```python
from build123d import *

# Parameters (mm, degrees)
SKETCH2_W           = 57
SKETCH2_H           = 37
BOSS_EXTRUDE1_DEPTH = 1.4
SKETCH1_R           = 1.35
CUT_EXTRUDE2_DEPTH  = 2.4
FILLET1_R           = 2
FILLET2_R           = 2
SKETCH4_R           = 2.5
SKETCH4_R_2         = 1.35
BOSS_EXTRUDE2_DEPTH = 1
CUT_EXTRUDE3_DEPTH  = 2.4


with BuildPart() as part:
    # Sketch2 → Boss-Extrude1 (new body)
    with BuildSketch(Plane(origin=(0, 0, 0), x_dir=(1, 0, 0), z_dir=(0, 1, 0))):
        Polygon((-27.5, -37.5), (-27.5, 37.5), (-22.5, 37.5), (-22.5, 23.5), (13.713455262, 23.5), (24.418761806, 38.487429162), (28.487429162, 35.581238194), (19.85797331, 23.5), (39.5, 23.5), (39.5, -23.5), (19.85797331, -23.5), (28.487429162, -35.581238194), (24.418761806, -38.487429162), (13.713455262, -23.5), (-22.5, -23.5), (-22.5, -37.5), align=None)
        with Locations((6, 0)):
            Rectangle(SKETCH2_W, SKETCH2_H, mode=Mode.SUBTRACT)
    extrude(amount=BOSS_EXTRUDE1_DEPTH)

    # Sketch1 → Cut-Extrude2 (cut, through all)
    with BuildSketch(Plane(origin=(0, 0, 0), x_dir=(1, 0, 0), z_dir=(0, 1, 0))):
        with Locations((-25, 35)):
            Circle(SKETCH1_R)
        with Locations((25, 35)):
            Circle(SKETCH1_R)
        with Locations((25, -35)):
            Circle(SKETCH1_R)
        with Locations((-25, -35)):
            Circle(SKETCH1_R)
        with Locations((-25, 21)):
            Circle(SKETCH1_R)
        with Locations((37, 21)):
            Circle(SKETCH1_R)
        with Locations((37, -21)):
            Circle(SKETCH1_R)
        with Locations((-25, -21)):
            Circle(SKETCH1_R)
    extrude(amount=CUT_EXTRUDE2_DEPTH, mode=Mode.SUBTRACT)

    # Fillet1
    fillet1_edges = [part.edges().sort_by_distance(p)[0] for p in [
        (28.487429162, 0.7, 35.581238194),
        (24.418761806, 0.7, 38.487429162),
        (-22.5, 0.7, 37.5),
        (-27.5, 0.7, 37.5),
        (-27.5, 0.7, -37.5),
        (-22.5, 0.7, -37.5),
        (24.418761806, 0.7, -38.487429162),
        (28.487429162, 0.7, -35.581238194),
    ]]
    fillet(fillet1_edges, radius=FILLET1_R)

    # Fillet2
    fillet2_edges = [part.edges().sort_by_distance(p)[0] for p in [
        (13.713455262, 0.7, 23.5),
        (-22.5, 0.7, 23.5),
        (-22.5, 0.7, -23.5),
        (13.713455262, 0.7, -23.5),
        (19.85797331, 0.7, -23.5),
        (19.85797331, 0.7, 23.5),
        (-22.5, 0.7, 18.5),
        (34.5, 0.7, 18.5),
        (34.5, 0.7, -18.5),
        (-22.5, 0.7, -18.5),
    ]]
    fillet(fillet2_edges, radius=FILLET2_R)

    # Sketch4 → Boss-Extrude2 (add)
    with BuildSketch(Plane(origin=(0, 1.4, 0), x_dir=(1, 0, 0), z_dir=(0, 1, 0))):
        with Locations((37, 21)):
            Circle(SKETCH4_R)
        with Locations((37, 21)):
            Circle(SKETCH4_R_2, mode=Mode.SUBTRACT)
        with Locations((37, -21)):
            Circle(SKETCH4_R)
        with Locations((37, -21)):
            Circle(SKETCH4_R_2, mode=Mode.SUBTRACT)
        with Locations((-25, -21)):
            Circle(SKETCH4_R)
        with Locations((-25, -21)):
            Circle(SKETCH4_R_2, mode=Mode.SUBTRACT)
        with Locations((-25, 21)):
            Circle(SKETCH4_R)
        with Locations((-25, 21)):
            Circle(SKETCH4_R_2, mode=Mode.SUBTRACT)
    extrude(amount=BOSS_EXTRUDE2_DEPTH)

    # Sketch5 → Cut-Extrude3 (cut, through all)
    with BuildSketch(Plane(origin=(0, 1.4, 0), x_dir=(1, 0, 0), z_dir=(0, 1, 0))):
        with BuildLine():
            Line((37, -23.5), (39.5, -23.5))
            Line((39.5, -23.5), (39.5, -21))
            ThreePointArc((39.5, -21), (38.767766953, -22.767766953), (37, -23.5))
        make_face()
        with BuildLine():
            Line((39.5, 21), (39.5, 23.5))
            Line((39.5, 23.5), (37, 23.5))
            ThreePointArc((37, 23.5), (38.767766953, 22.767766953), (39.5, 21))
        make_face()
    extrude(amount=-CUT_EXTRUDE3_DEPTH, mode=Mode.SUBTRACT)


solid = part.part
```
Input: part model. Units: mm. Frame: model coordinates. A direction names the side the tool comes from. Coordinates: 2 decimals unless noted, no trailing zeros. Write each loop counter-clockwise with the first axis right and the second up, starting at its lowest first coordinate (ties: lowest second). Pieces come first, ordered by that corner, then holes.
1) Section A-A on z = 9.5. Output: boundary loops of the cut face in (x, y), and give its area (3 significant figures).
2) Section C-C on x = 25. Output: boundary loops of the cut face in (y, z).
3) Section B-B on x = 1.5. Output: boundary loops of the cut face in (y, z).
4) Set-up query: faces 4 (the cylindrical face through (-23.1, 0.71, 36.93)), 5 (the flat face through (-23.9, 2.4, -19.9)), 6 (the cylindrical face through (-21.93, 0.71, -17.9)), 7 (the flat face through (24.684, 0.69, 30.257)), 8 (the cylindrical face through (-23.1, 0.71, -36.93)). Return all of +Z, -Z, +X, -X, +Y, -Y with unobstructed straight access to the full face (end or side cutting, diameter ignored); none if empty.
5) Mould query, pull axis X, two halves, no side actions, for faces 1 (the cylindrical face through (-26.93, 0.71, 36.9)), 2 (the flat face through (4, 0, 19)), 3 (the cylindrical face through (25.62, 0.69, 36.2)). Classes: pulls with the +X half, pulls with the -X half, needs draft (parallel to the pull), parting line crosses it, or undercut.
6) Material intervals for line 1 along Z through (x, y) = (37, 1.7); line 2 along Z through (x, y) = (-25, 0.35); line 3 along X through (y, z) = (1.9, -21), sorted ascending.
7) Pin query (flat end, axial travel): pin 1 Ø1.1 at (x, y) = (29, 0.5) entering from -Z; pin 2 Ø0.8 at (x, y) = (-25, 1) entering from +Z; pin 3 Ø8 at (x, z) = (16.5, 11) entering from +Y; pin 4 Ø0.8 at (x, y) = (-25, 0.5) entering from -Z. Return the tip coordinate at first contact, or that it passes through.
Check result:
1. outline: (-27.5, 0) - (-22.5, 0) - (-22.5, 1.4) - (-27.5, 1.4) - close; (34.5, 0) - (39.5, 0) - (39.5, 1.4) - (34.5, 1.4) - close
1. area: 14.0 mm2
2. outline: (0, -37.69) - (1.4, -37.69) - (1.4, -36.35) - (0, -36.35) - close; (0, -33.65) - (1.4, -33.65) - (1.4, -30.7) - (0, -30.7) - close; (0, -23.5) - (1.4, -23.5) - (1.4, -18.5) - (0, -18.5) - close; (0, 18.5) - (1.4, 18.5) - (1.4, 23.5) - (0, 23.5) - close; (0, 30.7) - (1.4, 30.7) - (1.4, 33.65) - (0, 33.65) - close; (0, 36.35) - (1.4, 36.35) - (1.4, 37.69) - (0, 37.69) - close
3. outline: (0, -23.5) - (1.4, -23.5) - (1.4, -18.5) - (0, -18.5) - close; (0, 18.5) - (1.4, 18.5) - (1.4, 23.5) - (0, 23.5) - close
4. face 4: +Z, +Y, -Y
4. face 5: +Z, -Z, +X, -X, +Y
4. face 6: +Y, -Y
4. face 7: +X, +Y, -Y
4. face 8: -Z, +Y, -Y
5. face 1: pulls with the -X half
5. face 2: needs draft
5. face 3: undercut
6. line 1: z = -23.5 to -22.35, -19.65 to -18.5, 18.5 to 19.65, 22.35 to 23.5
6. line 2: z = -37.5 to -36.35, -33.65 to -22.35, -19.65 to 19.65, 22.35 to 33.65, 36.35 to 37.5
6. line 3: x = -27.5 to -26.35, -23.65 to -22.5, 34.5 to 35.65, 38.35 to 39.5
7. pin 1: stops at z = -23.5
7. pin 2: stops at z = 37.5
7. pin 3: passes through
7. pin 4: stops at z = -37.5
